The drawing under review shows one solid part. Ordinate dimensions are in mm from its lowest x, y, z. A direction names the side the tool comes from. Give positions to 0.01 mm unless a question says otherwise; leave off trailing zeros. Loops run counter-clockwise (first coordinate to the right, second up) from the corner with the lowest first, then second, coordinate; pieces in that order, holes last. Notation, with made-up numbers: (-12.75, 68.5) -> (24.25, 68.5) arc R35 ccw to (24.25, 101.5) -> close; hole circle Ø2 at (-2, 46.5). An arc over 180 degrees is marked (long way). Answer in a Markdown table with one row per item. Add a question column.
(1) For line 1 (X direction, y = 19.75, z = 15.25); line 2 (Z direction, x = 49.5, y = 14.75), list the stretches that pass through material, from the lowest coordinate up.
(2) Consider section A-A on z = 12. Write out the cut boundary in (x, y), then the cut area to 3 significant figures.
(3) Consider section D-D on z = 4.5. Write out the cut boundary in (x, y), then the cut area to 3 significant figures.
(4) For pin 1 (5 mm diameter, centred on x = 57, y = 13, fed in from -Z); pin 2 (3 mm diameter, centred on x = 60.5, z = 16.5, fed in from +Y), all flat-tipped, find the tip position at first contact; note any pin that passes through.
(5) For the marked faces 1 and 2, list the 3-axis set-ups (+Z, -Z, +X, -X, +Y, -Y) from which the entire face can be reached by the end or side of a thin tool; tool diameter is ignored.
(6) Draft analysis for pull direction X (two halves, no side actions). For the marked faces 3, 4 and 5, state which applies: +X half, -X half, draft (parallel to the pull), parting line (faces both ways), or undercut.
(7) Consider section C-C on x = 11.5. Write out the cut boundary in (y, z).
(8) Consider section B-B on y = 17.5. Write out the cut boundary in (x, z).
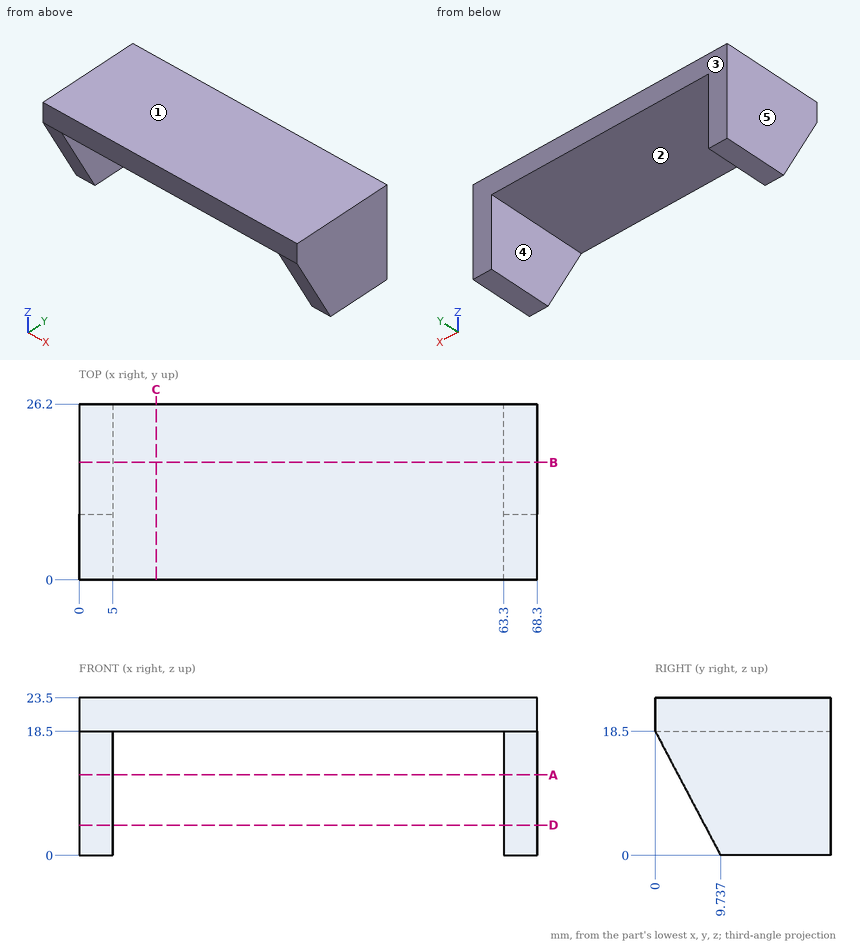
Values follow:
| question | item | result |
|---|---|---|
| 1 | line 1 | 0 to 5, 63.3 to 68.3 |
| 1 | line 2 | 18.5 to 23.5 |
| 2 | outline | (0, 3.42) -> (5, 3.42) -> (5, 26.2) -> (0, 26.2) -> close; (63.3, 3.42) -> (68.3, 3.42) -> (68.3, 26.2) -> (63.3, 26.2) -> close |
| 2 | area | 228 mm2 |
| 3 | outline | (0, 7.37) -> (5, 7.37) -> (5, 26.2) -> (0, 26.2) -> close; (63.3, 7.37) -> (68.3, 7.37) -> (68.3, 26.2) -> (63.3, 26.2) -> close |
| 3 | area | 188 mm2 |
| 4 | pin 1 | z = 18.5 |
| 4 | pin 2 | through |
| 5 | face 1 | +Z, +X, -X, +Y, -Y |
| 5 | face 2 | -Z, +Y, -Y |
| 6 | face 3 | draft |
| 6 | face 4 | undercut |
| 6 | face 5 | -X half |
| 7 | outline | (0, 18.5) -> (26.2, 18.5) -> (26.2, 23.5) -> (0, 23.5) -> close |
| 8 | outline | (0, 0) -> (5, 0) -> (5, 18.5) -> (63.3, 18.5) -> (63.3, 0) -> (68.3, 0) -> (68.3, 23.5) -> (0, 23.5) -> close |
